from build123d import *

# Parameters (mm, degrees)
SKETCH_R        = 10
SKETCH_R_2      = 3.1
SKETCH_R_3      = 2.5
PAD_DEPTH       = 15
SKETCH001_R     = 5.4
POCKET_DEPTH    = 6.5
SKETCH002_R     = 12.4
POCKET001_DEPTH = 6.2


with BuildPart() as part:
    # Sketch → Pad (new body)
    with BuildSketch(Plane(origin=(0, 0, 0), x_dir=(0, -1, 0), z_dir=(-1, 0, 0))):
        Polygon((-60, 0), (60, 0), (60, -42), (40, -58.4), (-40, -58.4), (-60, -42), align=None)
        with Locations((0, -37.5)):
            Circle(SKETCH_R, mode=Mode.SUBTRACT)
        with Locations((-36, -21.5)):
            Circle(SKETCH_R_2, mode=Mode.SUBTRACT)
        with Locations((36, -21.5)):
            Circle(SKETCH_R_2, mode=Mode.SUBTRACT)
        with Locations((49, -37.5)):
            Circle(SKETCH_R_3, mode=Mode.SUBTRACT)
        with Locations((-49, -37.5)):
            Circle(SKETCH_R_3, mode=Mode.SUBTRACT)
    extrude(amount=PAD_DEPTH)

    # Sketch001 → Pocket (cut)
    with BuildSketch(Plane(origin=(-15, 0, 0), x_dir=(0, -1, 0), z_dir=(-1, 0, 0))):
        with Locations((-36, -21.5)):
            Circle(SKETCH001_R)
        with Locations((36, -21.5)):
            Circle(SKETCH001_R)
    extrude(amount=-POCKET_DEPTH, mode=Mode.SUBTRACT)

    # Sketch002 → Pocket001 (cut)
    with BuildSketch(Plane(origin=(-15, 0, 0), x_dir=(0, -1, 0), z_dir=(-1, 0, 0))):
        with Locations((0, -37.5)):
            Circle(SKETCH002_R)
    extrude(amount=-POCKET001_DEPTH, mode=Mode.SUBTRACT)


solid = part.part
Check sheet for the modelled part. Datum: model origin and axes. Units: mm. A direction names the side the tool comes from. Coordinates: 2 decimals unless noted, no trailing zeros. Loops run counter-clockwise (first coordinate to the right, second up) from the corner with the lowest first, then second, coordinate; pieces in that order, holes last. Notation, with made-up numbers: (21.5, -38) -> (57.5, -38) arc R26 cw to (57.5, -15) -> close; hole circle Ø4 at (-21, -18.5). An arc over 180 degrees is marked (long way). Answer in a Markdown table with one row per item.
1. Sectioned sample at D-D, the plane z = -21.5. Record the boundary of the cut face in (x, y), then the cut area to 3 significant figures.
Check values:
| item | result |
|---|---|
| outline | (-15, -60) -> (0, -60) -> (0, -39.1) -> (-8.5, -39.1) -> (-8.5, -41.4) -> (-15, -41.4) -> close; (-15, -30.6) -> (-8.5, -30.6) -> (-8.5, -32.9) -> (0, -32.9) -> (0, 32.9) -> (-8.5, 32.9) -> (-8.5, 30.6) -> (-15, 30.6) -> close; (-15, 41.4) -> (-8.5, 41.4) -> (-8.5, 39.1) -> (0, 39.1) -> (0, 60) -> (-15, 60) -> close |
| area | 1,550 mm2 |
2. Sectioned sample at C-C, the plane x = -11. Record the boundary of the cut face in (y, z), then the cut area to 3 significant figures.
Check values:
| item | result |
|---|---|
| outline | (-60, -42) -> (-40, -58.4) -> (40, -58.4) -> (60, -42) -> (60, 0) -> (-60, 0) -> close; hole circle Ø5 at (-49, -37.5); hole circle Ø10.8 at (-36, -21.5); hole circle Ø24.8 at (0, -37.5); hole circle Ø10.8 at (36, -21.5); hole circle Ø5 at (49, -37.5) |
| area | 5,970 mm2 |
3. Go/stop test with flat-tipped pins: pin 1 (7 mm diameter, centred on y = -36, z = -21.5, fed in from -X); pin 2 (12 mm diameter, centred on y = 0, z = -37.5, fed in from -X); pin 3 (7.5 mm diameter, centred on y = -6, z = -35.5, fed in from -X). Record where each tip stops, or that it passes through.
Check values:
| item | result |
|---|---|
| pin 1 | stops at x = -8.5 |
| pin 2 | passes through |
| pin 3 | stops at x = -8.8 |
4. Sectioned sample at B-B, the plane z = -37.5. Record the boundary of the cut face in (x, y).
Check values:
| item | result |
|---|---|
| outline | (-15, -60) -> (0, -60) -> (0, -51.5) -> (-15, -51.5) -> close; (-15, -46.5) -> (0, -46.5) -> (0, -10) -> (-8.8, -10) -> (-8.8, -12.4) -> (-15, -12.4) -> close; (-15, 12.4) -> (-8.8, 12.4) -> (-8.8, 10) -> (0, 10) -> (0, 46.5) -> (-15, 46.5) -> close; (-15, 51.5) -> (0, 51.5) -> (0, 60) -> (-15, 60) -> close |
5. Sectioned sample at A-A, the plane y = -49. Record the boundary of the cut face in (x, z), then the cut area to 3 significant figures.
Check values:
| item | result |
|---|---|
| outline | (-15, -51.02) -> (0, -51.02) -> (0, -40) -> (-15, -40) -> close; (-15, -35) -> (0, -35) -> (0, 0) -> (-15, 0) -> close |
| area | 690 mm2 |
6. Material ranges on line 1 along Z through (x, y) = (-5, 36); line 2 along Y through (x, z) = (-9, -20.5); line 3 along Z through (x, y) = (-13.25, 36), recorded low to high. Write a range as [from, to].
Check values:
| item | result |
|---|---|
| line 1 | z = [-58.4, -24.6], [-18.4, 0] |
| line 2 | y = [-60, -41.31], [-30.69, 30.69], [41.31, 60] |
| line 3 | z = [-58.4, -26.9], [-16.1, 0] |
7. Release check for a two-part mould opening along Y. For faces 3 (the face through (-7.395, -50.14, -50.085)), 4 (the face through (-15, -1, -22)), 5 (the face through (-11.8, -41.15, -19.88)) record: released by +Y, released by -Y, zero draft, split by the parting line, or undercut.
Check values:
| item | result |
|---|---|
| face 3 | released by -Y |
| face 4 | zero draft |
| face 5 | undercut |
8. Access from +Z, -Z, +X, -X, +Y, -Y to the whole of each face (thin tool, end or side, straight path). Record for faces 1 (the face through (-8.5, -38.3, -23.8)), 2 (the face through (-4.34, 2.17, -47.26)).
Check values:
| item | result |
|---|---|
| face 1 | -X |
| face 2 | +X, -X |
